```python
from build123d import *

# Parameters (mm, degrees)
SKETCH1_W             = 40
SKETCH1_H             = 33
BOSS_EXTRUDE1_DEPTH   = 4
SKETCH3_W             = 40
SKETCH3_H             = 3
BOSS_EXTRUDE2_DEPTH   = 39.2
SKETCH10_W            = 2
SKETCH10_H            = 7.5
BOSS_EXTRUDE3_DEPTH   = 27.3
SKETCH12_W            = 4
SKETCH12_H            = 33
BOSS_EXTRUDE4_DEPTH   = 5
SKETCH13_W            = 2.5
SKETCH13_H            = 8
CUT_EXTRUDE5_DEPTH    = 50.856193196
CUT_EXTRUDE6_REACH    = 63.565
SKETCH15_R            = 1.75
FILLET6_R             = 3.75
CUT_EXTRUDE8_REACH    = 51.856
SKETCH23_R            = 1.25
FILLET8_R             = 2
SKETCH25_R            = 1
CUT_EXTRUDE10_DEPTH   = 59.234354122
SKETCH26_W            = 8
SKETCH26_H            = 2.5
CUT_EXTRUDE11_DEPTH   = 50.856193196
FILLET3_R             = 0.25
FILLET6_OF_MIRROR10_R = 3.75
FILLET8_OF_MIRROR10_R = 2
SKETCH28_W            = 8
SKETCH28_H            = 2.5
CUT_EXTRUDE12_DEPTH   = 50.856193196
FILLET9_R             = 0.25
CHAMFER1_SIZE         = 1.5
CHAMFER1_SIZE_2       = 4.121216129
CHAMFER2_SIZE         = 9.470627272
CHAMFER2_SIZE_2       = 1.5
SKETCH29_W            = 15
SKETCH29_H            = 15
CUT_EXTRUDE13_DEPTH   = 5
FILLET10_R            = 1.5


# Some blends are built 0.0001 mm under size
with BuildPart() as part:
    # Sketch1 → Boss-Extrude1 (new body)
    with BuildSketch(Plane.XY):
        with Locations((0, -1.5)):
            Rectangle(SKETCH1_W, SKETCH1_H)
    extrude(amount=BOSS_EXTRUDE1_DEPTH)

    # Sketch3 → Boss-Extrude2 (add)
    with BuildSketch(Plane.XY.offset(4)):
        with Locations((0, 13.5)):
            Rectangle(SKETCH3_W, SKETCH3_H)
    extrude(amount=BOSS_EXTRUDE2_DEPTH)

    # Sketch10 → Boss-Extrude3 (add)
    with BuildSketch(Plane.XZ.offset(-12)):
        with Locations((19, 39.45)):
            Rectangle(SKETCH10_W, SKETCH10_H)
    boss_extrude3 = extrude(amount=BOSS_EXTRUDE3_DEPTH)

    # Sketch12 → Boss-Extrude4 (add)
    with BuildSketch(Plane(origin=(20, 0, 0), x_dir=(0, 0, -1), z_dir=(1, 0, 0))):
        with Locations((-2, -1.5)):
            Rectangle(SKETCH12_W, SKETCH12_H)
    boss_extrude4 = extrude(amount=BOSS_EXTRUDE4_DEPTH)

    # Sketch13 → Cut-Extrude5 (cut, through all)
    with BuildSketch(Plane.XY.offset(4)):
        with Locations((20.75, -11.475)):
            Rectangle(SKETCH13_W, SKETCH13_H)
    cut_extrude5 = extrude(amount=-CUT_EXTRUDE5_DEPTH, mode=Mode.SUBTRACT)

    # Sketch15 → Cut-Extrude6 (cut, up to next)
    with BuildSketch(Plane(origin=(20, 0, 0), x_dir=(0, 0, -1), z_dir=(1, 0, 0)), mode=Mode.PRIVATE) as cut_extrude6_sk1:
        with Locations((-39.45, -11.475)):
            Circle(SKETCH15_R)
    cut_extrude6_tool1 = extrude(cut_extrude6_sk1.sketch, amount=-CUT_EXTRUDE6_REACH, mode=Mode.PRIVATE) & part.part
    cut_extrude6 = cut_extrude6_tool1.solids().sort_by_distance((20, -11.475, 39.45))[0]
    add(cut_extrude6, mode=Mode.SUBTRACT)

    # Fillet6
    fillet6_edges = [part.edges().sort_by_distance(p)[0] for p in [
        (19, -15.3, 35.7),
        (19, -15.3, 43.2),
    ]]
    fillet(fillet6_edges, radius=FILLET6_R - 0.0001)  # a hair under: the kernel refuses the full size

    # Sketch23 → Cut-Extrude8 (cut, up to next)
    with BuildSketch(Plane.XY.offset(4), mode=Mode.PRIVATE) as cut_extrude8_sk1:
        with Locations((11.4, -12.5)):
            Circle(SKETCH23_R)
    cut_extrude8_tool1 = extrude(cut_extrude8_sk1.sketch, amount=-CUT_EXTRUDE8_REACH, mode=Mode.PRIVATE) & part.part
    # Sketch23 → Cut-Extrude8 (cut, up to next)
    with BuildSketch(Plane.XY.offset(4), mode=Mode.PRIVATE) as cut_extrude8_sk2:
        with Locations((22.5, 12.5)):
            Circle(SKETCH23_R)
    cut_extrude8_tool2 = extrude(cut_extrude8_sk2.sketch, amount=-CUT_EXTRUDE8_REACH, mode=Mode.PRIVATE) & part.part
    cut_extrude8_1 = cut_extrude8_tool1.solids().sort_by_distance((11.4, -12.5, 4))[0]
    add(cut_extrude8_1, mode=Mode.SUBTRACT)
    cut_extrude8_2 = cut_extrude8_tool2.solids().sort_by_distance((22.5, 12.5, 4))[0]
    add(cut_extrude8_2, mode=Mode.SUBTRACT)
    cut_extrude8 = cut_extrude8_1 + cut_extrude8_2  # Cut-Extrude8 as one shape, for the pattern or mirror that repeats it

    # Fillet8
    fillet8_edges = [part.edges().sort_by_distance(p)[0] for p in [
        (25, 15, 2),
        (25, -18, 2),
    ]]
    fillet(fillet8_edges, radius=FILLET8_R)

    # Sketch25 → Cut-Extrude10 (cut, through all)
    with BuildSketch(Plane.XZ.offset(-12)):
        with Locations(Location((6, 39.45, 0), (0, 0, 270))):
            Circle(SKETCH25_R)
        with Locations(Location((-8, 39.45, 0), (0, 0, 270))):
            Circle(SKETCH25_R)
    extrude(amount=-CUT_EXTRUDE10_DEPTH, mode=Mode.SUBTRACT)

    # Sketch26 → Cut-Extrude11 (cut, through all)
    with BuildSketch(Plane.XY.offset(4)):
        with Locations((6, 5.75)):
            Rectangle(SKETCH26_W, SKETCH26_H)
    extrude(amount=-CUT_EXTRUDE11_DEPTH, mode=Mode.SUBTRACT)

    # Fillet3
    fillet3_edges = [part.edges().sort_by_distance(p)[0] for p in [
        (22, -7.475, 2),
        (22, -15.475, 2),
        (19.5, -15.475, 2),
        (19.5, -7.475, 2),
    ]]
    fillet(fillet3_edges, radius=FILLET3_R)

    # Mirror10: Boss-Extrude3, Boss-Extrude4, Cut-Extrude5, Cut-Extrude6, Cut-Extrude8 across plane
    add(boss_extrude3.mirror(Plane(origin=(0, 0, 0), x_dir=(0, 0, 1), z_dir=(1, 0, 0))))
    add(boss_extrude4.mirror(Plane(origin=(0, 0, 0), x_dir=(0, 0, 1), z_dir=(1, 0, 0))))
    add(cut_extrude5.mirror(Plane(origin=(0, 0, 0), x_dir=(0, 0, 1), z_dir=(1, 0, 0))), mode=Mode.SUBTRACT)
    add(cut_extrude6.mirror(Plane(origin=(0, 0, 0), x_dir=(0, 0, 1), z_dir=(1, 0, 0))), mode=Mode.SUBTRACT)
    add(cut_extrude8.mirror(Plane(origin=(0, 0, 0), x_dir=(0, 0, 1), z_dir=(1, 0, 0))), mode=Mode.SUBTRACT)

    # Fillet6 of Mirror10
    fillet6_of_mirror10_edges = [part.edges().sort_by_distance(p)[0] for p in [
        (-19, -15.3, 35.7),
        (-19, -15.3, 43.2),
    ]]
    fillet(fillet6_of_mirror10_edges, radius=FILLET6_OF_MIRROR10_R - 0.0001)  # a hair under: the kernel refuses the full size

    # Fillet8 of Mirror10
    fillet8_of_mirror10_edges = [part.edges().sort_by_distance(p)[0] for p in [
        (-25, 15, 2),
        (-25, -18, 2),
    ]]
    fillet(fillet8_of_mirror10_edges, radius=FILLET8_OF_MIRROR10_R)

    # Sketch28 → Cut-Extrude12 (cut, through all)
    with BuildSketch(Plane.XY.offset(4)):
        with Locations((-8, 5.75)):
            Rectangle(SKETCH28_W, SKETCH28_H)
    extrude(amount=-CUT_EXTRUDE12_DEPTH, mode=Mode.SUBTRACT)

    # Fillet9
    fillet9_edges = [part.edges().sort_by_distance(p)[0] for p in [
        (10, 4.5, 2),
        (2, 4.5, 2),
        (-12, 4.5, 2),
        (-4, 4.5, 2),
    ]]
    fillet(fillet9_edges, radius=FILLET9_R)

    # Chamfer1
    # the kernel refuses this chamfer: 4.121216129, 1.5 mm, written as the material it takes off along each edge
    with BuildSketch(Plane(origin=(-12, 4.75, 4), x_dir=(-0.9950833631817486, 0, 0.09904090225205062), z_dir=(0, 1, 0)), Plane(origin=(-4, 7, 4), x_dir=(0.9950833631817486, 0, 0.09904090225205064), z_dir=(0, -1, 0))) as chamfer1_piece_1:
        Polygon((CHAMFER1_SIZE * 0.995083363182, -CHAMFER1_SIZE * 0.0990409022521), (-CHAMFER1_SIZE_2 * 0.0990409022564, -CHAMFER1_SIZE_2 * 0.995083363226), (0, 0), align=None)
    extrude(amount=2.25, mode=Mode.SUBTRACT)
    with BuildSketch(Plane(origin=(-11.75, 4.75, 4), x_dir=(-1, 0, 0), z_dir=(0, 1, 0))) as chamfer1_piece_2:
        Polygon((0.25 + CHAMFER1_SIZE, 0), (0.25, -CHAMFER1_SIZE_2), (0.25, 0), align=None)
    revolve(axis=Axis((-11.75, 4.75, 4), (0, 0, 1)), revolution_arc=90, mode=Mode.SUBTRACT)
    with BuildSketch(Plane(origin=(-4.25, 4.75, 4), x_dir=(0, -1, 0), z_dir=(-1, 0, 0))) as chamfer1_piece_3:
        Polygon((0.25 + CHAMFER1_SIZE, 0), (0.25, -CHAMFER1_SIZE_2), (0.25, 0), align=None)
    revolve(axis=Axis((-4.25, 4.75, 4), (0, 0, 1)), revolution_arc=90, mode=Mode.SUBTRACT)
    with BuildSketch(Plane(origin=(-4.25, 4.5, 4), x_dir=(0, -0.9950833631817486, 0.09904090225205064), z_dir=(-1, 0, 0))) as chamfer1_piece_4:
        Polygon((CHAMFER1_SIZE * 0.995083363182, -CHAMFER1_SIZE * 0.0990409022521), (-CHAMFER1_SIZE_2 * 0.0990409022564, -CHAMFER1_SIZE_2 * 0.995083363226), (0, 0), align=None)
    extrude(amount=7.5, mode=Mode.SUBTRACT)

    # Chamfer2
    # the kernel refuses this chamfer: 9.470627272, 1.5 mm, written as the material it takes off along each edge
    with BuildSketch(Plane(origin=(2, 7, 0), x_dir=(0.006019451551713046, 0, 0.9999818829373942), z_dir=(0, -1, 0)), Plane(origin=(10, 4.75, 0), x_dir=(-0.006019451551713001, 0, 0.9999818829373942), z_dir=(0, 1, 0))) as chamfer2_piece_1:
        Polygon((CHAMFER2_SIZE * 0.999981882939, CHAMFER2_SIZE * 0.00601945155172), (-CHAMFER2_SIZE_2 * 0.00601945155171, CHAMFER2_SIZE_2 * 0.999981882937), (0, 0), align=None)
    extrude(amount=2.25, mode=Mode.SUBTRACT)
    with BuildSketch(Plane(origin=(2.25, 4.75, 0), x_dir=(-1, 0, 0), z_dir=(0, 1, 0))) as chamfer2_piece_2:
        Polygon((0.25, CHAMFER2_SIZE), (0.25 + CHAMFER2_SIZE_2, 0), (0.25, 0), align=None)
    revolve(axis=Axis((2.25, 4.75, 0), (0, 0, 1)), revolution_arc=90, mode=Mode.SUBTRACT)
    with BuildSketch(Plane(origin=(9.75, 4.75, 0), x_dir=(1, 0, 0), z_dir=(0, 1, 0))) as chamfer2_piece_3:
        Polygon((0.25, -CHAMFER2_SIZE), (0.25 + CHAMFER2_SIZE_2, 0), (0.25, 0), align=None)
    revolve(axis=Axis((9.75, 4.75, 0), (0, 0, -1)), revolution_arc=90, mode=Mode.SUBTRACT)
    with BuildSketch(Plane(origin=(2.25, 4.5, 0), x_dir=(0, 0.006019451551713091, 0.9999818829373942), z_dir=(1, 0, 0))) as chamfer2_piece_4:
        Polygon((CHAMFER2_SIZE * 0.999981882939, CHAMFER2_SIZE * 0.00601945155172), (-CHAMFER2_SIZE_2 * 0.00601945155171, CHAMFER2_SIZE_2 * 0.999981882937), (0, 0), align=None)
    extrude(amount=7.5, mode=Mode.SUBTRACT)

    # Sketch29 → Cut-Extrude13 (cut)
    with BuildSketch(Plane(origin=(0, 15, 0), x_dir=(1, 0, 0), z_dir=(0, 1, 0))):
        with Locations((0, -7.5)):
            Rectangle(SKETCH29_W, SKETCH29_H)
    extrude(amount=-CUT_EXTRUDE13_DEPTH, mode=Mode.SUBTRACT)

    # Fillet10
    fillet10_edges = [part.edges().sort_by_distance(p)[0] for p in [
        (-7.5, 10, 2),
        (-7.5, 13.5, 15),
        (7.5, 10, 2),
        (7.5, 13.5, 15),
    ]]
    fillet(fillet10_edges, radius=FILLET10_R)


solid = part.part
```
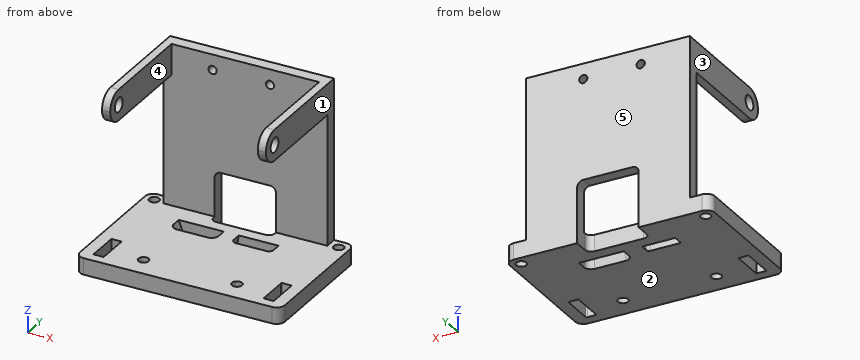
Source: CAD feature listing. Evaluate the final solid. Frame: model axes, mm. Face numbers are marked on the shaded views. A direction names the side the tool comes from. Give positions to 0.01 mm unless a question says otherwise; leave off trailing zeros. Loops run counter-clockwise (first coordinate to the right, second up) from the corner with the lowest first, then second, coordinate; pieces in that order, holes last. Notation, with made-up numbers: (52.5, 36.5) - (69.5, 36.5) arc R13 cw to (69.5, 56.5) - close; hole circle Ø3 at (15.5, -39.75). An arc over 180 degrees is marked (long way). Use CSV: the item, a comma, the result in double quotes.
1) Cut plane C-C (x = 15). Output: boundary loops of the cut face in (y, z).
Worked out:
outline,"(-18, 0) - (15, 0) - (15, 43.2) - (12, 43.2) - (12, 4) - (-18, 4) - close"
2) Line query: line 1 (X direction, y = 13.05, z = 39.45); line 2 (Y direction, x = 11, z = 2); line 3 (X direction, y = 10.5, z = 37). Output: solid intervals per line, ascending.
Worked out:
line 1,"x = -20 to -9, -7 to 5, 7 to 20"
line 2,"y = -18 to -13.68, -11.32 to 4.05, 7 to 15"
line 3,"x = -20 to -18, 18 to 20"
3) Cut plane B-B (x = -5). Output: boundary loops of the cut face in (y, z), and give its area (3 significant figures).
Worked out:
outline,"(-18, 0) - (4.46, 0) - (3, 4) - (-18, 4) - close; (7, 0) - (10, 0) - (10, 4) - (7, 4) - close; (12, 15) - (15, 15) - (15, 43.2) - (12, 43.2) - close"
area,"184 mm^2"
4) Set-up query: the marked faces 1, 2, 3, 4 and 5. Return all of +Z, -Z, +X, -X, +Y, -Y with unobstructed straight access to the full face (end or side cutting, diameter ignored); none if empty.
Worked out:
face 1,"+Z, +X, +Y, -Y"
face 2,"-Z, +X, -X, +Y, -Y"
face 3,"+Z, -X, +Y, -Y"
face 4,"+Z, -Y"
face 5,"+Z, -Z, +X, -X, +Y"
5) Pin query (flat end, axial travel): P1, Ø3, axis at x = -12, z = 27.5, coming from the -Y side; P2, Ø3, axis at x = 22.5, y = 12.5, coming from the +Z side; P3, Ø2, axis at y = -4.5, z = 40.5, coming from the +X side. Return the tip coordinate at first contact, or that it passes through.
Worked out:
P1,"stops at y = 12"
P2,"stops at z = 4"
P3,"stops at x = 20"
6) Cut plane D-D (z = 21.5). Output: boundary loops of the cut face in (x, y).
Worked out:
outline,"(-20, 12) - (20, 12) - (20, 15) - (-20, 15) - close"
7) Cut plane A-A (z = 11). Output: boundary loops of the cut face in (x, y).
Worked out:
outline,"(-20, 12) - (-7.5, 12) - (-7.5, 15) - (-20, 15) - close; (7.5, 12) - (20, 12) - (20, 15) - (7.5, 15) - close"
